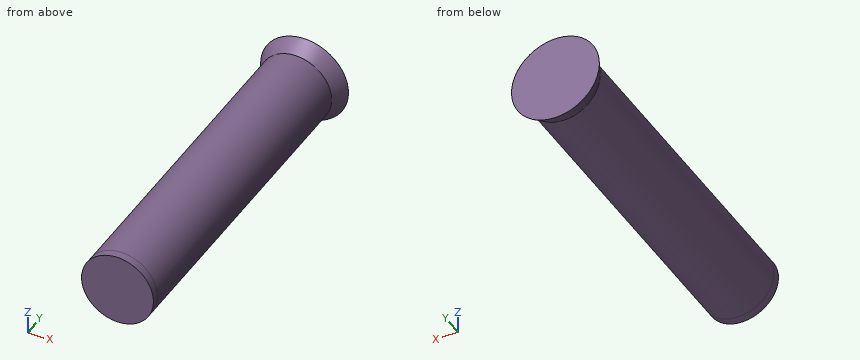
```python
from build123d import *

# Parameters (mm, degrees)
SKETCH1_R           = 9
BOSS_EXTRUDE1_DEPTH = 80
BOSS_EXTRUDE2_START = 2
SKETCH2_R           = 9
BOSS_EXTRUDE2_DEPTH = 2


with BuildPart() as part:
    # Sketch1 → Boss-Extrude1 (new body)
    with BuildSketch(Plane(origin=(0, 0, 0), x_dir=(1, 0, 0), z_dir=(0, 1, 0))):
        with Locations(Location((0, 0, 0), (0, 0, 270))):
            Circle(SKETCH1_R)
    extrude(amount=BOSS_EXTRUDE1_DEPTH)

    # Sketch2 → Boss-Extrude2 (add)
    with BuildSketch(Plane.XZ.offset(BOSS_EXTRUDE2_START)):
        with Locations(Location((0, 0, 0), (0, 0, 270))):
            Circle(SKETCH2_R)
    extrude(amount=-BOSS_EXTRUDE2_DEPTH)

    # Sketch4 → Revolve1 (revolve)
    with BuildSketch(Plane(origin=(0, 0, 0), x_dir=(0, 0, -1), z_dir=(1, 0, 0))):
        Polygon((9, 80), (0, 80), (0, 84.007892879), (11, 84.007892879), align=None)
    revolve(axis=Axis((0, 75.015231433, 0), (0, 1, 0)))


solid = part.part
```
Build history of the part. All positions in model axes, mm. Give positions to 0.01 mm unless a question says otherwise; leave off trailing zeros. Loops run counter-clockwise (first coordinate to the right, second up) from the corner with the lowest first, then second, coordinate; pieces in that order, holes last. Notation, with made-up numbers: (-34, 83.25) -> (8, 83.25) arc R12 cw to (8, 89.25) -> close; hole circle Ø11 at (-16, 79.5). An arc over 180 degrees is marked (long way). One line per question, with ' | ' between items.
Q1. Cut at B-B, the plane z = 0. Write the cut outline in (x, y).
Filled sheet:
outline: (-11, 84.01) -> (-9, 80) -> (-9, -2) -> (9, -2) -> (9, 80) -> (11, 84.01) -> close
Q2. Drop flat-ended pins along their axis: pin 1 (8 mm diameter, centred on x = -2, y = 16, fed in from +Z); pin 2 (6 mm diameter, centred on x = 6, y = 73, fed in from +Z); pin 3 (5 mm diameter, centred on y = 10, z = -7.5, fed in from +X). Give the stop position or say it passes through.
Filled sheet:
pin 1: stops at z = 9 | pin 2: stops at z = 8.49 | pin 3: stops at x = 7.48
Q3. Drill centre lines: line 1 along X through (y, z) = (28, 0.5); line 2 along X through (y, z) = (40, -7); line 3 along Y through (x, z) = (9.25, -1). Where is each one in solid material? Low to high. Write a range as [from, to].
Filled sheet:
line 1: x = [-8.99, 8.99] | line 2: x = [-5.66, 5.66] | line 3: y = [80.61, 84.01]
Q4. Cut at A-A, the plane x = 0. Write the cut outline in (y, z), plus the area to 3 significant figures.
Filled sheet:
outline: (-2, -9) -> (80, -9) -> (84.01, -11) -> (84.01, 11) -> (80, 9) -> (-2, 9) -> close | area: 1,560 mm²
Q5. Cut at C-C, the plane y = 13.5. Write the cut outline in (x, z).
Filled sheet:
outline: circle Ø18 at (0, 0)
